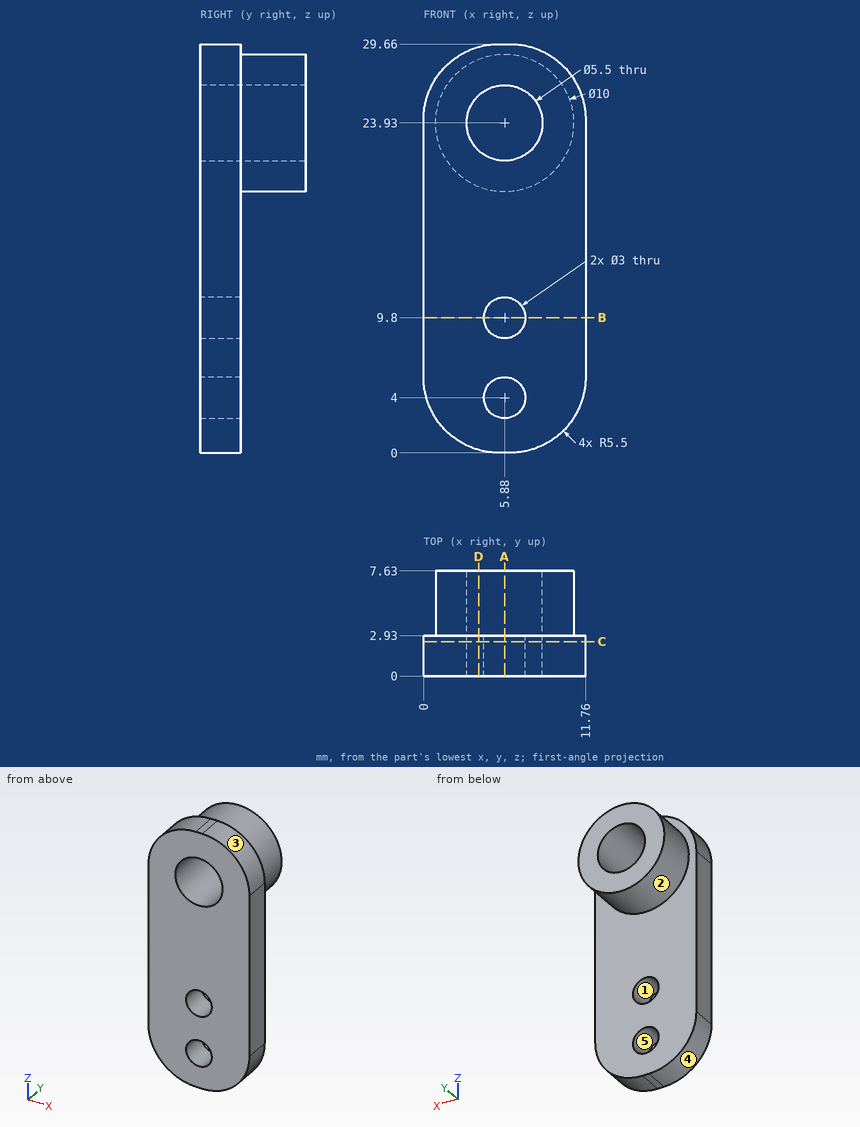
Input: dimensioned drawing with shaded views. Units: mm. Origin: part minimum x, y, z. A direction names the side the tool comes from. Round coordinates to 2 decimals unless told otherwise and drop trailing zeros. Order: outer loops, then holes, each group sorted by start corner. A loop starts at its lowest first (then second) coordinate and runs counter-clockwise, first axis right, second up. Notation, with made-up numbers: (-17, 7) - (12, 7) arc R31 ccw to (12, 35) - close; hole circle Ø3 at (-11.75, -9.75). An arc over 180 degrees is marked (long way). Answer as a JSON object with one key per item and string values. Group by question number.
(1) Material intervals for probe 1 along X at (y, z) = (1.35, 9.8); probe 2 along X at (y, z) = (2, 23.93); probe 3 along Z at (x, y) = (5.25, 1.5), sorted ascending. Write a range as from..to.
(2) Cut plane A-A (x = 5.88). Return loops of the section in (y, z).
(3) Cut plane C-C (y = 2.5). Return loops of the section in (x, z), then the cut area to 3 significant figures.
(4) Draft query along X for the marked faces 3, 4 and 5. Return one class per face: released by +X, released by -X, zero draft, split by the parting line, or undercut.
(5) Reachability of the marked faces 1 and 2 from +Z, -Z, +X, -X, +Y, -Y: full face, straight path, thin tool, end or side. Return the list, or none.
(6) Cut plane D-D (x = 4). Return loops of the section in (y, z), then the cut area to 3 significant figures.
(7) Cut plane B-B (z = 9.8). Return loops of the section in (x, y).
(8) Pin query (flat end, axial travel): P1, Ø1.5, axis at x = 3, y = 5, coming from the +Z side; P2, Ø2, axis at x = 10, y = 1, coming from the +Z side; P3, Ø2, axis at y = 4, z = 13, coming from the +X side. Return the tip coordinate at first contact, or that it passes through.
Here are the results:
{
 "1": {"probe 1": "x = 0..4.38, 7.38..11.76", "probe 2": "x = 0..3.13, 8.63..11.76", "probe 3": "z = 0.01..2.64, 5.36..8.44, 11.16..21.25, 26.61..29.65"},
 "2": {"outline": "(0, 0) - (2.93, 0) - (2.93, 2.5) - (0, 2.5) - close; (0, 5.5) - (2.93, 5.5) - (2.93, 8.3) - (0, 8.3) - close; (0, 11.3) - (2.93, 11.3) - (2.93, 18.93) - (7.63, 18.93) - (7.63, 21.18) - (0, 21.18) - close; (0, 26.68) - (7.63, 26.68) - (7.63, 28.93) - (2.93, 28.93) - (2.93, 29.66) - (0, 29.66) - close"},
 "3": {"outline": "(0, 5.5) arc R5.5 ccw to (5.5, 0) - (6.26, 0) arc R5.5 ccw to (11.76, 5.5) - (11.76, 24.16) arc R5.5 ccw to (6.26, 29.66) - (5.5, 29.66) arc R5.5 ccw to (0, 24.16) - close; hole circle Ø5.5 at (5.88, 23.93); hole circle Ø3 at (5.88, 4); hole circle Ø3 at (5.88, 9.8)", "area": "285 mm^2"},
 "4": {"face 3": "released by +X", "face 4": "released by -X", "face 5": "undercut"},
 "5": {"face 1": "+Y, -Y", "face 2": "+Y"},
 "6": {"outline": "(0, 0.21) - (2.93, 0.21) - (2.93, 19.3) - (7.63, 19.3) - (7.63, 21.92) - (0, 21.92) - close; (0, 25.94) - (7.63, 25.94) - (7.63, 28.56) - (2.93, 28.56) - (2.93, 29.45) - (0, 29.45) - close", "area": "98.6 mm^2"},
 "7": {"outline": "(0, 0) - (4.38, 0) - (4.38, 2.93) - (0, 2.93) - close; (7.38, 0) - (11.76, 0) - (11.76, 2.93) - (7.38, 2.93) - close"},
 "8": {"P1": "stops at z = 28.45", "P2": "stops at z = 28.93", "P3": "passes through"}
}
